For this review, take the finished solid that the model builds, in its own axes (mm). Face numbers are marked on the shaded views. A direction names the side the tool comes from. Round coordinates to 2 decimals unless told otherwise and drop trailing zeros. Loops run counter-clockwise (first coordinate to the right, second up) from the corner with the lowest first, then second, coordinate; pieces in that order, holes last.
Autodesk Fusion 360 part; units mm, degrees
sketch "Switch" plane through (0, 0, 0) normal (0, 0, 1) x (1, 0, 0)
  line L0 (0, 0) -> (148, 0)
  line L1 (148, 0) -> (148, 100)
  line L2 (148, 100) -> (0, 100)
  line L3 (0, 100) -> (0, 0)
  line L4 (-3, 100) -> (7, 100)
  line L5 (7, 100) -> (7, -3)
  line L6 (7, -3) -> (-3, -3)
  line L7 (-3, -3) -> (-3, 100)
  line L8 (-3, 100) -> (-18, 100)
  line L9 (-18, 100) -> (-18, 85)
  line L10 (-18, 85) -> (-3, 85)
  line L11 (-3, 85) -> (-3, 100)
  line L12 (-3, -3) -> (-18, -3)
  line L13 (-18, -3) -> (-18, 12)
  line L14 (-18, 12) -> (-3, 12)
  line L15 (-3, 12) -> (-3, -3)
  circle A0 centre (-10.5, 5.75) radius 2
  circle A1 centre (-10.5, 91.25) radius 2
  line L16 (-3, -3) -> (-18, -3)
  line L17 (-18, -3) -> (-18, -0.5)
  line L18 (-18, -0.5) -> (-3, -0.5)
  line L19 (-3, -0.5) -> (-3, -3)
  line L20 (-3, 100) -> (-18, 100)
  line L21 (-18, 100) -> (-18, 97.5)
  line L22 (-18, 97.5) -> (-3, 97.5)
  line L23 (-3, 97.5) -> (-3, 100)
  dimension "d1" = 100
  dimension "d2" = 148
  dimension "d3" = 7
  dimension "d4" = 3
  dimension "d6" = 3
  dimension "d7" = 15
  dimension "d8" = 15
  dimension "d10" = 15
  dimension "d12" = 4
  dimension "d13" = 4
  dimension "d21" = 7.5
  dimension "d31" = 6.25
  dimension "d32" = 15
  dimension "d33" = 2.5
  dimension "d34" = 7.5
  dimension "d35" = 2.5
  dimension "d36" = 6.25
extrude "Extrude1" add sketch "Switch" along normal blind 33.5 contours L0 L3 L4 L5 L6 L7 L11 L15 L19 L23
extrude "Extrude2" add sketch "Switch" along normal blind 2.5 from surface at 31 contours L0 L2 L3 L4 L5
extrude "Extrude3" add sketch "Switch" along normal blind 2.5 contours L7 L9 L10 L11 L22 | L7 L13 L14 L15 L18
extrude "Extrude5" add sketch "Switch" along normal blind 18 contours L7 L8 L9 L11 L20 L21 L22 L23 | L7 L12 L13 L15 L16 L17 L18 L19
sketch "Venting hole" plane through (0, 0, 0) normal (1, 0, 0) x (0, 1, 0)
  line L0 (92.5, 8.3) -> (6.5, 8.3)
  line L1 (6.5, 8.3) -> (6.5, 21.3)
  line L2 (6.5, 21.3) -> (92.5, 21.3)
  line L3 (92.5, 21.3) -> (92.5, 8.3)
  line L4 (0, 0) -> (0, 31)
  line L5 (100, 0) -> (100, 18)
  point P0 (100, 0)
  dimension "d40" = 8.3
  dimension "d41" = 6.5
  dimension "d42" = 7.5
  dimension "d43" = 13
extrude "Extrude6" cut sketch "Venting hole" against normal blind 10
fillet "Fillet1" radius 4 4 edges at (-1.5, 6.5, 21.3) (-1.5, 6.5, 8.3) (-1.5, 92.5, 8.3) (-1.5, 92.5, 21.3)
fillet "Fillet2" radius 3 2 edges at (2, -3, 33.5) (2, 100, 33.5)
chamfer "Chamfer1" distance 15 angle 45 2 edges at (-18, 98.75, 18) (-18, -1.75, 18)
fillet "Fillet3" radius 3 2 edges at (-18, 12, 1.25) (-18, 85, 1.25)
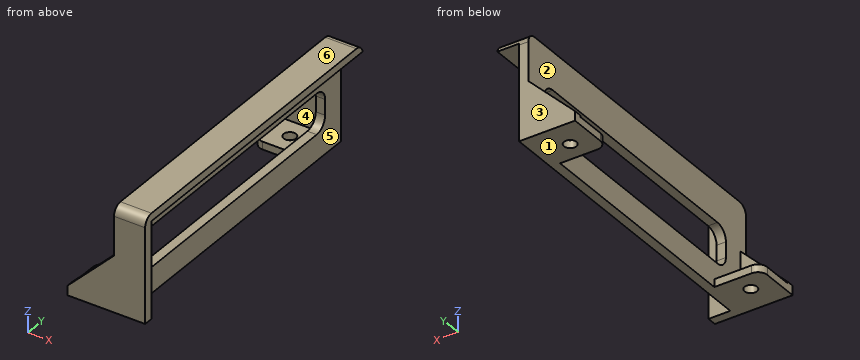
(1) For L1, parallel to Y at x = -10.5, z = 0.8; L2, parallel to Y at x = -5.75, z = 15; L3, parallel to Z at x = 3.25, y = 74.5, list the stretches that pass through material, from the lowest coordinate up.
(2) Add section C-C (x = -4). Give the boundary of the cut face in (y, z).
(3) Add section B-B (z = 19). Give the boundary of the cut face in (x, y), plus the area to 3 significant figures.
(4) Insertion check: pin 1 Ø4.5 at (x, y) = (-10.5, 5.75) entering from +Z; pin 2 Ø1 at (x, z) = (-7.5, 16) entering from -Y; pin 3 Ø3 at (x, y) = (3.5, 49) entering from -Z; pin 4 Ø5 at (y, z) = (79, 27) entering from +X. Each pin has a flat end and moves straight along its axis. Give the tip position at first contact, or say it passes through.
(5) Add section A-A (y = 91.25). Give the boundary of the cut face in (x, z), plus the area to 3 significant figures.
(6) Add section D-D (y = 51.5). Give the boundary of the cut face in (x, z).
(7) The part is to be moulded in two halves that separate along Y. For the marked faces 1, 2 and 3, say which applies: pulls with the +Y half, pulls with the -Y half, needs draft (parallel to the pull), parting line crosses it, or undercut.
(8) For the marked faces 4, 5 and 6, list the 3-axis set-ups (+Z, -Z, +X, -X, +Y, -Y) from which the entire face can be reached by the end or side of a thin tool; tool diameter is ignored.
Outcome:
1. L1: y = -3 to 3.75, 7.75 to 12, 85 to 89.25, 93.25 to 100
1. L2: y = -3 to -0.5, 97.5 to 100
1. L3: z = 31 to 33.5
2. outline: (-3, 0) - (12, 0) - (12, 2.5) - (-0.5, 2.5) - (-0.5, 17) - (-3, 17) - close; (85, 0) - (100, 0) - (100, 17) - (97.5, 17) - (97.5, 2.5) - (85, 2.5) - close
3. outline: (-3, -3) - (7, -3) - (7, 0) - (0, 0) - (0, 6.88) - (-3, 6.88) - close; (-3, 92.12) - (0, 92.12) - (0, 100) - (-3, 100) - close
3. area: 74.3 mm2
4. pin 1: stops at z = 2.5
4. pin 2: passes through
4. pin 3: stops at z = 31
4. pin 4: stops at x = 0
5. outline: (-18, 0) - (-12.5, 0) - (-12.5, 2.5) - (-18, 2.5) - close; (-8.5, 0) - (0, 0) - (0, 9.4) - (-3, 9.4) - (-3, 2.5) - (-8.5, 2.5) - close; (-3, 20.2) - (0, 20.2) - (0, 31) - (7, 31) - (7, 33.5) - (-3, 33.5) - close
5. area: 113 mm2
6. outline: (-3, 0) - (0, 0) - (0, 8.3) - (-3, 8.3) - close; (-3, 21.3) - (0, 21.3) - (0, 31) - (7, 31) - (7, 33.5) - (-3, 33.5) - close
7. face 1: needs draft
7. face 2: undercut
7. face 3: pulls with the +Y half
8. face 4: +Z, -X
8. face 5: -Z, +X, +Y
8. face 6: +Z, +X, -X, +Y, -Y
